from build123d import *

# Parameters (mm, degrees)
F1_DEPTH  = 2
F3_DEPTH  = 1.5
F5_W      = 4
F5_H      = 5.5
F6_DEPTH  = 52
F4_R      = 1.25
F7_DEPTH  = 5
F8_W      = 1.5
F8_H      = 10.6
F9_DEPTH  = 25
F11_DEPTH = 2


with BuildPart() as f1:
    # F0 (on Top) → F1 (new body)
    with BuildSketch(Plane.XY):
        Polygon((-32.848224, 11.779634), (-32.848224, 6.779634), (-24.848224, 6.779634), (-24.848224, 11.779634), (-26.848224, 13.779634), (-30.848224, 13.779634), align=None)
    extrude(amount=F1_DEPTH)

    # F2 (on face) → F3 (join)
    with BuildSketch(Plane.XZ.offset(-6.779634)):
        Polygon((-32.848224, 5), (-32.848224, 2), (-24.848224, 2), (-24.848224, 5), (-26.848224, 7), (-26.848224, 49), (-24.848224, 51), (-24.848224, 56), (-32.848224, 56), (-32.848224, 51), (-30.848224, 49), (-30.848224, 7), align=None)
    extrude(amount=-F3_DEPTH)

    # F5 (on face) → F6 (join)
    with BuildSketch(Plane.XY.offset(2)):
        with Locations((-28.848224, 11.029634)):
            Rectangle(F5_W, F5_H)
    extrude(amount=F6_DEPTH)

    # F4 (on face) → F7 (cut)
    with BuildSketch(Plane.XZ.offset(-6.779634)):
        with Locations((-28.848224, 5)):
            Circle(F4_R)
        with Locations((-28.848224, 51)):
            Circle(F4_R)
    extrude(amount=-F7_DEPTH, mode=Mode.SUBTRACT)

    # F8 (on face) → F9 (cut)
    with BuildSketch(Plane(origin=(-30.848224, 0, 0), x_dir=(0, -1, 0), z_dir=(-1, 0, 0))):
        with Locations((-9.029634, 13.75)):
            Rectangle(F8_W, F8_H)
        with Locations((-9.029634, 34.05)):
            Rectangle(F8_W, F8_H)
    extrude(amount=-F9_DEPTH, mode=Mode.SUBTRACT)

    # F10 (on face) → F11 (join)
    with BuildSketch(Plane.XY.offset(56)):
        Polygon((-32.848224, 8.279634), (-24.848224, 8.279634), (-24.848224, 11.779634), (-26.893736, 13.779634), (-30.893736, 13.779634), (-32.848224, 11.779634), align=None)
    extrude(amount=-F11_DEPTH)


solid = f1.part
CAD build for the part. Positions are in the model's coordinates, mm. A direction names the side the tool comes from. Round coordinates to 2 decimals unless told otherwise and drop trailing zeros. Order: outer loops, then holes, each group sorted by start corner. A loop starts at its lowest first (then second) coordinate and runs counter-clockwise, first axis right, second up. Notation, with made-up numbers: (73.25, 53.25) -> (84.25, 53.25) arc R29 ccw to (84.25, 86.25) -> close; hole circle Ø9 at (16, 28.25). An arc over 180 degrees is marked (long way). Write item = value, one per line. Start each with the question number.
(1) Which spindle directions (+Z, -Z, +X, -X, +Y, -Y) get a long thin tool onto all of the face, cutting with end or side? Do faces 1 (the flat face through (-29, 11.78, 5)), 2 (the flat face through (-29, 9.78, 34)), 3 (the flat face through (-32, 8.28, 4)), 4 (the flat face through (-31.86, 7.52, 50.01)), 5 (the flat face through (-26, 8.28, 4)). Say none if no direction does.
(2) Pull direction X, two halves, no side cores. Call faces 6 (the flat face through (-31.86, 12.79, 55.01)), 7 (the flat face through (-24.848, 9, 55)), 8 (the flat face through (-29, 11.78, 51)), 9 (the cylindrical face through (-29.01, 9.24, 52.24)): released by +X, released by -X, zero draft, split by the parting line, or undercut.
(3) Cut at A-A, the plane y = 8.75. List the corners of the cut face in (x, z), then the cut area to 3 significant figures.
(4) Probe line 1 (Y direction, x = -27, z = 38); line 2 (Z direction, x = -30.75, y = 8.5); line 3 (Z direction, x = -25.75, y = 10.5). List the from-to ranges inside material, lowest first. Write a range as [from, to].
(5) Pin check, flat tips, straight feed: P1, Ø3.5, axis at y = 10.5, z = 16, coming from the +X side; P2, Ø1.2, axis at x = -29, z = 5.5, coming from the -Y side; P3, Ø1.6, axis at x = -32, z = 52, coming from the +Y side. Stop position of each tip, or through.
(6) Cut at B-B, the plane z = 10.5. List the corners of the cut face in (x, y), then the cut area to 3 significant figures.
(7) Cut at D-D, the plane z = 23.5. List the corners of the cut face in (x, y).
(8) Cut at C-C, the plane x = -26. List the corners of the cut face in (y, z), then the cut area to 3 significant figures.
Model answer:
q1.face_1 = -Y
q1.face_2 = +X, -X
q1.face_3 = -X, +Y
q1.face_4 = -X, +Y, -Y
q1.face_5 = +X, +Y
q2.face_6 = released by -X
q2.face_7 = released by +X
q2.face_8 = undercut
q2.face_9 = undercut
q3.outline = (-32.85, 0) -> (-24.85, 0) -> (-24.85, 2) -> (-26.85, 2) -> (-26.85, 8.45) -> (-30.85, 8.45) -> (-30.85, 2) -> (-32.85, 2) -> close; (-32.85, 54) -> (-30.85, 54) -> (-30.85, 39.35) -> (-26.85, 39.35) -> (-26.85, 54) -> (-24.85, 54) -> (-24.85, 56) -> (-32.85, 56) -> close; (-30.85, 19.05) -> (-26.85, 19.05) -> (-26.85, 28.75) -> (-30.85, 28.75) -> close; hole circle Ø2.5 at (-28.85, 5); hole circle Ø2.5 at (-28.85, 51)
q3.area = 145 mm2
q4.line_1 = [6.78, 8.28], [9.78, 13.78]
q4.line_2 = [0, 8.45], [19.05, 28.75], [39.35, 56]
q4.line_3 = [0, 2], [54, 56]
q5.P1 = -26.85
q5.P2 = 11.78
q5.P3 = 8.28
q6.outline = (-30.85, 6.78) -> (-26.85, 6.78) -> (-26.85, 8.28) -> (-30.85, 8.28) -> close; (-30.85, 9.78) -> (-26.85, 9.78) -> (-26.85, 13.78) -> (-30.85, 13.78) -> close
q6.area = 22.0 mm2
q7.outline = (-30.85, 6.78) -> (-26.85, 6.78) -> (-26.85, 13.78) -> (-30.85, 13.78) -> close
q8.outline = (6.78, 0) -> (12.93, 0) -> (12.93, 2) -> (8.28, 2) -> (8.28, 6.15) -> (6.78, 6.15) -> close; (6.78, 49.85) -> (8.28, 49.85) -> (8.28, 54) -> (12.91, 54) -> (12.91, 56) -> (6.78, 56) -> close
q8.area = 37.0 mm2
